```python
from build123d import *

# Parameters (mm, degrees)
ESBO_O1_R                  = 15
RESSALTO_EXTRUS_O1_DEPTH   = 25
ESBO_O2_R                  = 13.5
CORTE_EXTRUS_O1_DEPTH      = 10
CORTE_EXTRUS_O3_DEPTH      = 16
CORTE_EXTRUS_O3_DEPTH_BACK = 16


with BuildPart() as part:
    # Esboço1 → Ressalto-extrusão1 (new body)
    with BuildSketch(Plane(origin=(0, 0, 0), x_dir=(1, 0, 0), z_dir=(0, 1, 0))):
        Circle(ESBO_O1_R)
    extrude(amount=RESSALTO_EXTRUS_O1_DEPTH)

    # Esboço2 → Corte-extrusão1 (cut)
    with BuildSketch(Plane(origin=(0, 25, 0), x_dir=(1, 0, 0), z_dir=(0, 1, 0))):
        Circle(ESBO_O2_R)
    extrude(amount=-CORTE_EXTRUS_O1_DEPTH, mode=Mode.SUBTRACT)

    # Esboço4 → Corte-extrusão3 (cut, two sides)
    with BuildSketch(Plane(origin=(0, 0, 0), x_dir=(0, 0, -1), z_dir=(1, 0, 0))) as corte_extrus_o3_sk:
        with BuildLine():
            ThreePointArc((4, 10.97706773), (-5.3, 7.5), (4, 4.02293227))
            Line((4, 4.02293227), (4, 10.97706773))
        make_face()
    extrude(amount=CORTE_EXTRUS_O3_DEPTH, mode=Mode.SUBTRACT)
    extrude(corte_extrus_o3_sk.sketch, amount=-CORTE_EXTRUS_O3_DEPTH_BACK, mode=Mode.SUBTRACT)


solid = part.part
```
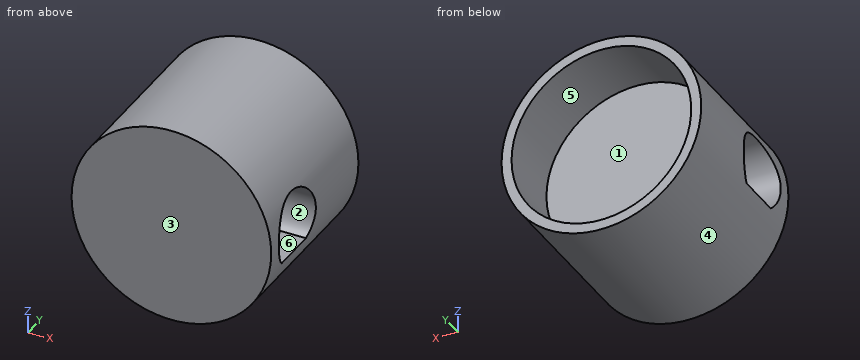
Model file for the job. Use its own axes, mm. Face numbers are marked on the shaded views. A direction names the side the tool comes from. Round coordinates to 2 decimals unless told otherwise and drop trailing zeros. Write each loop counter-clockwise with the first axis right and the second up, starting at its lowest first coordinate (ties: lowest second). Pieces come first, ordered by that corner, then holes. Notation, with made-up numbers: (-22.5, 25) - (30.5, 25) arc R18 cw to (30.5, 34) - close; hole circle Ø8 at (-7.75, -20). An arc over 180 degrees is marked (long way). Use CSV: the item, a comma, the result in double quotes. Start each with the question number.
Item 1: Tool access for the marked faces 4, 5 and 6: list every direction of +Z, -Z, +X, -X, +Y, -Y with a clear straight run to the whole face (end or side of a thin tool).
Item 2: Band-saw the part on B-B (x = 4.5). Write the cut outline in (y, z).
Item 3: Pin check, flat tips, straight feed: P1, Ø8.5, axis at y = 7.5, z = 0, coming from the +X side; P2, Ø4, axis at y = 12, z = 7, coming from the +X side; P3, Ø13.5, axis at x = 4, z = -1, coming from the +Y side. Stop position of each tip, or through.
Item 4: Band-saw the part on A-A (z = 0). Write the cut outline in (x, y).
Item 5: Drill centre lines: L1, parallel to Y at x = 4, z = 0; L2, parallel to Z at x = 0, y = 18.5. Where is each one in solid material? Low to high. Write a range as [from, to].
Item 6: Band-saw the part on D-D (z = -11). Write the cut outline in (x, y), and give its area (3 significant figures).
Item 7: Two-plate mould, pull along Y, no slides. Class the marked faces 1, 2 and 3: released by +Y, released by -Y, zero draft, split by the parting line, or undercut.
Item 8: Band-saw the part on C-C (y = 20). Write the cut outline in (x, z), and give its area (3 significant figures).
Checked values:
1,face 4,"+Y, -Y"
1,face 5,"+Y"
1,face 6,"+X, -X"
2,outline,"(0, -14.31) - (25, -14.31) - (25, -12.73) - (15, -12.73) - (15, 12.73) - (25, 12.73) - (25, 14.31) - (0, 14.31) - close; hole (4.02, -4) - (10.98, -4) arc R5.3 ccw (long way) to start"
3,P1,"stops at x = 14.46"
3,P2,"stops at x = 14.14"
3,P3,"stops at y = 15"
4,outline,"(-15, 0) - (15, 0) - (15, 2.2) - (-15, 2.2) - close; (-15, 12.8) - (15, 12.8) - (15, 25) - (13.5, 25) - (13.5, 15) - (-13.5, 15) - (-13.5, 25) - (-15, 25) - close"
5,L1,"y = [0, 2.2], [12.8, 15]"
5,L2,"z = [-15, -13.5], [13.5, 15]"
6,outline,"(-10.2, 0) - (10.2, 0) - (10.2, 25) - (7.83, 25) - (7.83, 15) - (-7.83, 15) - (-7.83, 25) - (-10.2, 25) - close"
6,area,"353 mm²"
7,face 1,"released by +Y"
7,face 2,"undercut"
7,face 3,"released by -Y"
8,outline,"circle Ø30 at (0, 0); hole circle Ø27 at (0, 0)"
8,area,"134 mm²"
